The listing builds one solid part. Answer for the finished solid, in the listing's coordinates (mm). A direction names the side the tool comes from. Give positions to 0.01 mm unless a question says otherwise; leave off trailing zeros. Loops run counter-clockwise (first coordinate to the right, second up) from the corner with the lowest first, then second, coordinate; pieces in that order, holes last. Notation, with made-up numbers: (62.5, 3) - (79.5, 3) arc R24 ccw to (79.5, 13) - close; hole circle Ø10 at (51, -25.75). An arc over 180 degrees is marked (long way). Write each question's results on one line, items separated by ' | '.
from build123d import *

# Parameters (mm, degrees)
BOSS_EXTRUDE1_START   = -31.115
BOSS_EXTRUDE1_DEPTH   = 62.23
BOSS_EXTRUDE1_2_DEPTH = 5.08
BOSS_EXTRUDE1_START_2 = 26.035
BOSS_EXTRUDE1_3_DEPTH = 5.08
SKETCH2_W             = 13.672898009
SKETCH2_H             = 52.07
CUT_EXTRUDE1_DEPTH    = 52.07
CUT_EXTRUDE3_DEPTH    = 51.80793688


with BuildPart() as part:
    # Boss-Extrude1: read off the stored shape, not the designer's step
    # Boss-Extrude1 outline → Boss-Extrude1 (new body)
    with BuildSketch(Plane(origin=(0, 0, 0), x_dir=(1, 0, 0), z_dir=(0, 1, 0)).offset(BOSS_EXTRUDE1_START)):
        with BuildLine():
            Line((-26.035, 12.7), (-26.035, -0.972898009))
            ThreePointArc((-26.035, -0.972898009), (-26.483762918, -0.272448114), (-27.269759251, 0))
            Line((-27.269759251, 0), (-31.115, 0))
            Line((-31.115, 0), (-31.115, -12.7))
            Line((-31.115, -12.7), (31.115, -12.7))
            Line((31.115, -12.7), (31.115, 12.7))
            Line((31.115, 12.7), (-26.035, 12.7))
        make_face()
    extrude(amount=BOSS_EXTRUDE1_DEPTH)

    # Boss-Extrude1 2 outline → Boss-Extrude1 2 (add)
    with BuildSketch(Plane(origin=(0, 0, 0), x_dir=(1, 0, 0), z_dir=(0, 1, 0)).offset(BOSS_EXTRUDE1_START)):
        with BuildLine():
            Line((-26.035, -0.972898009), (-26.035, 0))
            Line((-26.035, 0), (-27.269759251, 0))
            ThreePointArc((-27.269759251, 0), (-26.483762918, -0.272448114), (-26.035, -0.972898009))
        make_face()
    extrude(amount=BOSS_EXTRUDE1_2_DEPTH)

    # Boss-Extrude1 3 outline → Boss-Extrude1 3 (add)
    with BuildSketch(Plane(origin=(0, 0, 0), x_dir=(1, 0, 0), z_dir=(0, 1, 0)).offset(BOSS_EXTRUDE1_START_2)):
        with BuildLine():
            Line((-26.035, -0.972898009), (-26.035, 0))
            Line((-26.035, 0), (-27.269759251, 0))
            ThreePointArc((-27.269759251, 0), (-26.483762918, -0.272448114), (-26.035, -0.972898009))
        make_face()
    extrude(amount=BOSS_EXTRUDE1_3_DEPTH)

    # Sketch2 → Cut-Extrude1 (cut)
    with BuildSketch(Plane.ZY.offset(26.035)):
        with Locations((-5.863550996, 0)):
            Rectangle(SKETCH2_W, SKETCH2_H)
    extrude(amount=-CUT_EXTRUDE1_DEPTH, mode=Mode.SUBTRACT)

    # Sketch4 → Cut-Extrude3 (cut, through all)
    with BuildSketch(Plane.XY.offset(12.7)):
        with BuildLine():
            Line((15.875, 16.302284846), (15.875, 20.0025))
            Line((15.875, 20.0025), (-15.875, 20.0025))
            Line((-15.875, 20.0025), (-15.875, -20.0025))
            Line((-15.875, -20.0025), (15.875, -20.0025))
            Line((15.875, -20.0025), (15.875, -16.302284846))
            ThreePointArc((15.875, -16.302284846), (16.590655575, -14.294238532), (18.415, -13.191432873))
            ThreePointArc((18.415, -13.191432873), (20.239344425, -12.088627214), (20.955, -10.0805809))
            Line((20.955, -10.0805809), (20.955, 10.0805809))
            ThreePointArc((20.955, 10.0805809), (20.239344425, 12.088627214), (18.415, 13.191432873))
            ThreePointArc((18.415, 13.191432873), (16.590655575, 14.294238532), (15.875, 16.302284846))
        make_face()
    extrude(amount=-CUT_EXTRUDE3_DEPTH, mode=Mode.SUBTRACT)

    # Sketch5 → Cut-Revolve1 (revolve, cut)
    with BuildSketch(Plane(origin=(0, 0, 4.578168392), x_dir=(-1, 0, 0), z_dir=(0, 0, -1)), mode=Mode.PRIVATE) as cut_revolve1_sk:
        with BuildLine():
            Line((8.730963547, -31.115), (10.318463547, -31.115))
            Line((10.318463547, -31.115), (10.318463547, -20.0025))
            Line((10.318463547, -20.0025), (7.460963547, -20.0025))
            ThreePointArc((7.460963547, -20.0025), (8.358989159, -20.374474388), (8.730963547, -21.2725))
            Line((8.730963547, -21.2725), (8.730963547, -31.115))
        make_face()
    revolve(cut_revolve1_sk.sketch.rotate(Axis((-10.318463547, -31.115, 4.578168392), (0, 1, 0)), 270), axis=Axis((-10.318463547, -31.115, 4.578168392), (0, 1, 0)), mode=Mode.SUBTRACT)

    # Sketch6 → Cut-Revolve2 (revolve, cut)
    with BuildSketch(Plane(origin=(0, 0, 4.578168392), x_dir=(-1, 0, 0), z_dir=(0, 0, -1)), mode=Mode.PRIVATE) as cut_revolve2_sk:
        with BuildLine():
            Line((-11.905963547, -31.115), (-10.318463547, -31.115))
            Line((-10.318463547, -31.115), (-10.318463547, -20.0025))
            Line((-10.318463547, -20.0025), (-13.175963547, -20.0025))
            ThreePointArc((-13.175963547, -20.0025), (-12.277937935, -20.374474388), (-11.905963547, -21.2725))
            Line((-11.905963547, -21.2725), (-11.905963547, -31.115))
        make_face()
    revolve(cut_revolve2_sk.sketch.rotate(Axis((10.318463547, -31.115, 4.578168392), (0, 1, 0)), 180), axis=Axis((10.318463547, -31.115, 4.578168392), (0, 1, 0)), mode=Mode.SUBTRACT)

    # Sketch7 → Cut-Revolve3 (revolve, cut)
    with BuildSketch(Plane(origin=(0, 0, 4.578168392), x_dir=(-1, 0, 0), z_dir=(0, 0, -1)), mode=Mode.PRIVATE) as cut_revolve3_sk:
        with BuildLine():
            Line((7.460963547, 20.0025), (10.318463547, 20.0025))
            Line((10.318463547, 20.0025), (10.318463547, 31.115))
            Line((10.318463547, 31.115), (8.730963547, 31.115))
            Line((8.730963547, 31.115), (8.730963547, 21.2725))
            ThreePointArc((8.730963547, 21.2725), (8.358989159, 20.374474388), (7.460963547, 20.0025))
        make_face()
    revolve(cut_revolve3_sk.sketch.rotate(Axis((-10.318463547, 20.0025, 4.578168392), (0, 1, 0)), 180), axis=Axis((-10.318463547, 20.0025, 4.578168392), (0, 1, 0)), mode=Mode.SUBTRACT)

    # Sketch8 → Cut-Revolve4 (revolve, cut)
    with BuildSketch(Plane(origin=(0, 0, 4.578168392), x_dir=(-1, 0, 0), z_dir=(0, 0, -1)), mode=Mode.PRIVATE) as cut_revolve4_sk:
        with BuildLine():
            Line((-13.175963547, 20.0025), (-10.318463547, 20.0025))
            Line((-10.318463547, 20.0025), (-10.318463547, 31.115))
            Line((-10.318463547, 31.115), (-11.905963547, 31.115))
            Line((-11.905963547, 31.115), (-11.905963547, 21.2725))
            ThreePointArc((-11.905963547, 21.2725), (-12.277937935, 20.374474388), (-13.175963547, 20.0025))
        make_face()
    revolve(cut_revolve4_sk.sketch.rotate(Axis((10.318463547, 20.0025, 4.578168392), (0, 1, 0)), 180), axis=Axis((10.318463547, 20.0025, 4.578168392), (0, 1, 0)), mode=Mode.SUBTRACT)


solid = part.part
Item 1: Find the intervals of material crossed by line 1 along X through (y, z) = (5, 4.75) (3 decimals); line 2 along Y through (x, z) = (0.5, 3.5) (1 decimal); line 3 along Y through (x, z) = (-15.5, -8.5) (3 decimals), in increasing order. Write a range as [from, to].
Values found:
line 1: x = [-31.115, -15.875], [20.955, 31.115] | line 2: y = [-31.1, -20], [20, 31.1] | line 3: y = [-31.115, -26.035], [26.035, 31.115]
Item 2: A cutting plane is placed at C-C, the plane z = -7. Determine the outline of the cut face in (x, y) (3 decimals).
Values found:
outline: (-26.035, -31.115) - (31.115, -31.115) - (31.115, 31.115) - (-26.035, 31.115) - (-26.035, 26.035) - (26.035, 26.035) - (26.035, -26.035) - (-26.035, -26.035) - close
Item 3: For faces 4 (the face through (-26.035, -29, -6)), 5 (the face through (15.875, -18, 7)), 6 (the face through (8.85, 26.12, 3.97)), determine the directions among +Z, -Z, +X, -X, +Y, -Y from which every point of the face is accessible in a straight line to the end or side of a thin tool.
Values found:
face 4: -Z, -X, +Y, -Y | face 5: +Z, -Z | face 6: +Y, -Y
Item 4: Flat-ended cylindrical pins translate along their axes: P1, Ø5.5, axis at y = 27.5, z = -4, coming from the -X side (3 decimals); P2, Ø4, axis at x = -17.5, y = 16.5, coming from the -Z side; P3, Ø4, axis at x = -29, y = 14, coming from the -Z side. Find the tip coordinate at first contact, or state that the pin passes through.
Values found:
P1: stops at x = -26.035 | P2: stops at z = 0.97 | P3: stops at z = 0
Item 5: A cutting plane is placed at B-B, the plane x = -15. Determine the outline of the cut face in (y, z) (1 decimal).
Values found:
outline: (-31.1, -12.7) - (-26, -12.7) - (-26, 1) - (-20, 1) - (-20, 12.7) - (-31.1, 12.7) - close; (20, 1) - (26, 1) - (26, -12.7) - (31.1, -12.7) - (31.1, 12.7) - (20, 12.7) - close
Item 6: A cutting plane is placed at D-D, the plane x = -22.5. Determine the outline of the cut face in (y, z) (3 decimals).
Values found:
outline: (-31.115, -12.7) - (-26.035, -12.7) - (-26.035, 0.973) - (26.035, 0.973) - (26.035, -12.7) - (31.115, -12.7) - (31.115, 12.7) - (-31.115, 12.7) - close
Item 7: For a pull along Y with two mould halves and no side action, classify faces 1 (the face through (-15.875, 0, 7)), 2 (the face through (0, 31.115, 0)), 3 (the face through (31.115, 0, 0)) as released by +Y, released by -Y, zero draft, split by the parting line, or undercut.
Values found:
face 1: undercut | face 2: released by +Y | face 3: zero draft
Item 8: A cutting plane is placed at A-A, the plane y = -8. Determine the outline of the cut face in (x, z) (3 decimals).
Values found:
outline: (-31.115, 0) - (-27.27, 0) arc R1.27 ccw to (-26.035, 0.973) - (-15.875, 0.973) - (-15.875, 12.7) - (-31.115, 12.7) - close; (20.955, 0.973) - (26.035, 0.973) - (26.035, -12.7) - (31.115, -12.7) - (31.115, 12.7) - (20.955, 12.7) - close
